Could you check a few things on this model? Use its own coordinates, in mm. A direction names the side the tool comes from. Give positions to 0.01 mm unless a question says otherwise; leave off trailing zeros. Order: outer loops, then holes, each group sorted by start corner. A loop starts at its lowest first (then second) coordinate and runs counter-clockwise, first axis right, second up.
(1) If we mould it in two halves opening along X, with no side actions, what happens to faces 3 (the cylindrical face through (13.4, 20.69, -1.61)), 4 (the flat face through (30, 76.2, -2)), 5 (the flat face through (29.591, 58, -2))? For each: released by +X, released by -X, zero draft, split by the parting line, or undercut.
(2) On a 3-axis mill with a long thin cutter (end or side, diameter ignored), from which of +Z, -Z, +X, -X, +Y, -Y can I reach the whole of each face in a straight line? I mean faces 1 (the cylindrical face through (40.62, 38.24, -6.93)), 2 (the flat face through (35, 67.31, -7)). Say none if no direction works.
(3) Will these pins go through, and if not, where does the flat tip stop? pin 1 (1.6 mm diameter, centred on y = 19, z = -1, fed in from +X); pin 2 (16 mm diameter, centred on x = 9, y = 41.5, fed in from -Z) (3 decimals).
(4) Imagine slicing it at D-D, the plane y = 63. Write out the boundary of the cut face in (x, z) (3 decimals), then the cut area to 3 significant figures.
(5) If I drill on probe 1 along Y at (x, z) = (37, -0.5); probe 2 along Z at (x, y) = (24, 32) (3 decimals); probe 3 along X at (y, z) = (61.5, -1.25), over which ranges is the centre line in solid material (lowest first)?
(6) Imagine slicing it at C-C, the plane z = -7.25. Write out the boundary of the cut face in (x, y), then the cut area to 3 significant figures.
(7) Imagine slicing it at A-A, the plane z = -1.75. Write out the boundary of the cut face in (x, y).
(8) Imagine slicing it at B-B, the plane y = 30. Write out the boundary of the cut face in (x, z) (3 decimals).
from build123d import *

# Parameters (mm, degrees)
SKETCH1_W           = 29.591
SKETCH1_H           = 3.175
SKETCH1_R           = 6.604
BOSS_EXTRUDE1_DEPTH = 76.2
SKETCH2_R           = 4.191
CUT_EXTRUDE1_DEPTH  = 50.8
CUT_EXTRUDE2_START  = 8.89
SKETCH1_3_R         = 6.604
CUT_EXTRUDE2_DEPTH  = 19.05
CUT_EXTRUDE3_START  = 48.26
SKETCH1_5_R         = 6.604
CUT_EXTRUDE3_DEPTH  = 19.05
SKETCH3_R           = 2.54
CUT_EXTRUDE4_DEPTH  = 90.327145258
FILLET1_R           = 7.62
FILLET2_R           = 7.62


with BuildPart() as part:
    # Sketch1 → Boss-Extrude1 (new body)
    with BuildSketch(Plane(origin=(0, 0, 0), x_dir=(1, 0, 0), z_dir=(0, 1, 0))):
        with Locations((14.7955, 1.5875)):
            Rectangle(SKETCH1_W, SKETCH1_H)
        with BuildLine():
            Line((32.455996545, 3.175), (29.591, 3.175))
            Line((29.591, 3.175), (29.591, 0))
            Line((29.591, 0), (38.1, 0))
            ThreePointArc((38.1, 0), (34.862122609, 0.84822325), (32.455996545, 3.175))
        make_face()
        with Locations((38.1, 6.604)):
            Circle(SKETCH1_R)
    extrude(amount=BOSS_EXTRUDE1_DEPTH)

    # Sketch2 → Cut-Extrude1 (cut)
    with BuildSketch(Plane(origin=(0, 0, -3.175), x_dir=(-1, 0, 0), z_dir=(0, 0, -1))):
        with Locations((-17.399, 56.769)):
            Circle(SKETCH2_R)
        with Locations((-17.399, 19.431)):
            Circle(SKETCH2_R)
    extrude(amount=-CUT_EXTRUDE1_DEPTH, mode=Mode.SUBTRACT)

    # Sketch1_3 → Cut-Extrude2 (cut)
    with BuildSketch(Plane(origin=(0, 0, 0), x_dir=(1, 0, 0), z_dir=(0, 1, 0)).offset(CUT_EXTRUDE2_START)):
        with BuildLine():
            Line((32.455996545, 3.175), (29.591, 3.175))
            Line((29.591, 3.175), (29.591, 0))
            Line((29.591, 0), (38.1, 0))
            ThreePointArc((38.1, 0), (34.862122609, 0.84822325), (32.455996545, 3.175))
        make_face()
        with Locations((38.1, 6.604)):
            Circle(SKETCH1_3_R)
    extrude(amount=CUT_EXTRUDE2_DEPTH, mode=Mode.SUBTRACT)

    # Sketch1_5 → Cut-Extrude3 (cut)
    with BuildSketch(Plane(origin=(0, 0, 0), x_dir=(1, 0, 0), z_dir=(0, 1, 0)).offset(CUT_EXTRUDE3_START)):
        with Locations((38.1, 6.604)):
            Circle(SKETCH1_5_R)
        with BuildLine():
            Line((32.455996545, 3.175), (29.591, 3.175))
            Line((29.591, 3.175), (29.591, 0))
            Line((29.591, 0), (38.1, 0))
            ThreePointArc((38.1, 0), (34.862122609, 0.84822325), (32.455996545, 3.175))
        make_face()
    extrude(amount=CUT_EXTRUDE3_DEPTH, mode=Mode.SUBTRACT)

    # Sketch3 → Cut-Extrude4 (cut, through all)
    with BuildSketch(Plane(origin=(0, 76.2, 0), x_dir=(1, 0, 0), z_dir=(0, 1, 0))):
        with Locations(Location((38.1, 6.604, 0), (0, 0, 270))):
            Circle(SKETCH3_R)
    extrude(amount=-CUT_EXTRUDE4_DEPTH, mode=Mode.SUBTRACT)

    # Fillet1
    fillet1_edges = [part.edges().sort_by_distance(p)[0] for p in [
        (0, 0, -1.5875),
    ]]
    fillet(fillet1_edges, radius=FILLET1_R)

    # Fillet2
    fillet2_edges = [part.edges().sort_by_distance(p)[0] for p in [
        (0, 76.2, -1.5875),
    ]]
    fillet(fillet2_edges, radius=FILLET2_R)


solid = part.part
Answer block:
1. face 3: undercut
1. face 4: zero draft
1. face 5: released by +X
2. face 1: +Y, -Y
2. face 2: +Z, -Z, +X
3. pin 1: stops at x = 29.59
3. pin 2: stops at z = -3.175
4. outline: (0, -3.175) - (29.591, -3.175) - (29.591, 0) - (0, 0) - close
4. area: 94.0 mm2
5. probe 1: y = 0 to 8.89, 27.94 to 48.26, 67.31 to 76.2
5. probe 2: z = -3.175 to 0
5. probe 3: x = 0 to 29.59
6. outline: (31.53, 0) - (35.64, 0) - (35.64, 8.89) - (31.53, 8.89) - close; (31.53, 27.94) - (35.64, 27.94) - (35.64, 48.26) - (31.53, 48.26) - close; (31.53, 67.31) - (35.64, 67.31) - (35.64, 76.2) - (31.53, 76.2) - close; (40.56, 0) - (44.67, 0) - (44.67, 8.89) - (40.56, 8.89) - close; (40.56, 27.94) - (44.67, 27.94) - (44.67, 48.26) - (40.56, 48.26) - close; (40.56, 67.31) - (44.67, 67.31) - (44.67, 76.2) - (40.56, 76.2) - close
6. area: 314 mm2
7. outline: (0, 7.62) arc R7.62 ccw to (7.62, 0) - (42.58, 0) - (42.58, 8.89) - (29.59, 8.89) - (29.59, 27.94) - (42.58, 27.94) - (42.58, 48.26) - (29.59, 48.26) - (29.59, 67.31) - (42.58, 67.31) - (42.58, 76.2) - (7.62, 76.2) arc R7.62 ccw to (0, 68.58) - close; hole circle Ø8.38 at (17.4, 19.43); hole circle Ø8.38 at (17.4, 56.77)
8. outline: (0, -3.175) - (32.456, -3.175) arc R6.604 ccw (long way) to (38.1, 0) - (0, 0) - close; hole circle Ø5.08 at (38.1, -6.604)
